Verification items for the finished model (mm, model axes). A direction names the side the tool comes from. Round coordinates to 2 decimals unless told otherwise and drop trailing zeros. Loops run counter-clockwise (first coordinate to the right, second up) from the corner with the lowest first, then second, coordinate; pieces in that order, holes last. Notation, with made-up numbers: M -27,23.5 L 9,23.5 A22 ccw 9,37.5 Z; hole C 61,13.25 d11. An arc over 180 degrees is marked long. Write item = value, one per line. Start each with the question number.
from build123d import *

# Parameters (mm, degrees)
F0_R     = 25.4
F1_DEPTH = 6.35
F2_R     = 22.225
F3_DEPTH = 6.35
F4_R     = 8
F5_DEPTH = 12.701
F6_SIZE  = 1.27


with BuildPart() as f1:
    # F0 (on Front) → F1 (new body)
    with BuildSketch(Plane.XZ):
        Circle(F0_R)
    extrude(amount=F1_DEPTH)

    # F2 (on face) → F3 (join)
    with BuildSketch(Plane.XZ.offset(6.35)):
        Circle(F2_R)
    extrude(amount=F3_DEPTH)

    # F4 (on Front) → F5 (cut, through all)
    with BuildSketch(Plane.XZ):
        Circle(F4_R)
    extrude(amount=F5_DEPTH, mode=Mode.SUBTRACT)

    # F6
    f6_edges = [f1.edges().sort_by_distance(p)[0] for p in [
        (-25.4, -6.35, 0),
    ]]
    chamfer(f6_edges, length=F6_SIZE)


solid = f1.part
1. Section check C-C, the plane y = -11.75. Enter the section's corners in (x, z) (3 decimals), and give its area (3 significant figures).
2. Section check A-A, the plane x = 0. Enter the section's corners in (y, z) (3 decimals), and give its area (3 significant figures).
3. Mould release check, pull along Z, two halves, no side actions. Record for faces 3 (the cylindrical face through (-5.506, -2.504, -24.796)), 4 (the cylindrical face through (-1.73, -6.26, -7.81)), 5 (the flat face through (0, -12.7, -10)): pulls with the +Z half, pulls with the -Z half, needs draft (parallel to the pull), parting line crosses it, or undercut.
4. Gauge pin test, flat ends, axial feed: P1, Ø6, axis at x = 2.5, y = -10, coming from the -Z side (3 decimals); P2, Ø3, axis at x = -9.5, y = -10.5, coming from the +Z side; P3, Ø6, axis at y = -3.5, z = 20, coming from the +X side; P4, Ø4, axis at x = -12, z = 19, coming from the -Y side. Record the tip position at first contact, or that the pin passes through.
5. Tool access check on faces 1 (the flat face through (-6, 0, 6)), 2 (the cylindrical face through (21.199, -9.481, 6.676)). Record the directions out of +Z, -Z, +X, -X, +Y, -Y that give a thin tool (end or side, any length) a straight path to the whole face; none if there is none.
6. Section check D-D, the plane y = -2.75. Enter the section's corners in (x, z), and give its area (3 significant figures).
7. Section check B-B, the plane z = 0. Enter the section's corners in (x, y) (3 decimals).
8. Thickness scan on line 1 (Z direction, x = 5.5, y = -0.5); line 2 (X direction, y = -5.75, z = -4); line 3 (Z direction, x = 0, y = -7.25) (3 decimals). Record the ranges inside material, lowest first.
Computed values:
q1.outline = C 0,0 d44.45; hole C 0,0 d16
q1.area = 1,350 mm2
q2.outline = M -12.7,-22.225 L -6.35,-22.225 L -6.35,-24.13 L -5.08,-25.4 L 0,-25.4 L 0,-8 L -12.7,-8 Z; M -12.7,8 L 0,8 L 0,25.4 L -5.08,25.4 L -6.35,24.13 L -6.35,22.225 L -12.7,22.225 Z
q2.area = 400 mm2
q3.face_3 = parting line crosses it
q3.face_4 = undercut
q3.face_5 = needs draft
q4.P1 = -22.225
q4.P2 = 20.74
q4.P3 = 18.87
q4.P4 = -12.7
q5.face_1 = +Z, -Z, +X, -X, +Y
q5.face_2 = -Y
q6.outline = C 0,0 d50.8; hole C 0,0 d16
q6.area = 1,830 mm2
q7.outline = M -25.4,-5.08 L -24.13,-6.35 L -22.225,-6.35 L -22.225,-12.7 L -8,-12.7 L -8,0 L -25.4,0 Z; M 8,-12.7 L 22.225,-12.7 L 22.225,-6.35 L 24.13,-6.35 L 25.4,-5.08 L 25.4,0 L 8,0 Z
q8.line_1 = -24.8 to -5.81, 5.81 to 24.8
q8.line_2 = -24.4 to -6.93, 6.93 to 24.4
q8.line_3 = -22.225 to -8, 8 to 22.225
